Read the model definition and answer for the solid it produces. Units are mm, in the model's axes. A direction names the side the tool comes from. Give positions to 0.01 mm unless a question says otherwise; leave off trailing zeros. Loops run counter-clockwise (first coordinate to the right, second up) from the corner with the lowest first, then second, coordinate; pieces in that order, holes last. Notation, with made-up numbers: (62.25, -35) - (76.25, -35) arc R24 cw to (76.25, -7) - close; hole circle Ø7 at (-7.5, 44.5). An arc over 180 degrees is marked (long way). Use a Markdown table: item, result. Add a question column.
Item 1: For a pull along Y with two mould halves and no side action, classify faces 5 (the face through (7, 0, 2)), 6 (the face through (7, 11, 0)), 7 (the face through (8.475, 4.619, 2.465)) as +Y half, -Y half, draft (parallel to the pull), parting line (faces both ways), or undercut.
Item 2: Each of these flat-tipped pins is pushed along its axis until it touches: P1, Ø7.5, axis at x = 9, y = 8, coming from the -Z side; P2, Ø3, axis at y = 5.5, z = -6.5, coming from the -X side; P3, Ø4, axis at y = 3, z = 3, coming from the -X side; P4, Ø8, axis at y = 7.5, z = -4.5, coming from the +X side. Where does it stop, or does it pass through?
Item 3: A cutting plane is placed at A-A (x = 146.35). Determine the outline of the cut face in (y, z).
Item 4: A cutting plane is placed at D-D (z = -2.5). Determine the outline of the cut face in (x, y), plus the area to 3 significant figures.
Item 5: Consider probe 1 along Y at (x, z) = (146.35, 1.3); probe 2 along X at (y, z) = (14.75, 2); probe 3 along X at (y, z) = (14.5, 3.5). Determine where each line is inside the solid, lowest interval first. Write a range as [from, to].
Item 6: Which of the six approach directions +Z, -Z, +X, -X, +Y, -Y give full straight-line access (tool end or side, diameter ignored) to faces 1 (the face through (15, 17, 3)), 2 (the face through (137.7, 2, 4)), 3 (the face through (75.491, 0.007, -2.17)), 4 (the face through (145, 11, 0))?
Item 7: A cutting plane is placed at C-C (x = 41.5). Determine the outline of the cut face in (y, z), plus the area to 3 significant figures.
Item 8: A cutting plane is placed at B-B (y = 5.5). Determine the outline of the cut face in (x, z), plus the area to 3 significant figures.
from build123d import *

# Parameters (mm, degrees)
SKETCH_W     = 15
SKETCH_H     = 21
SKETCH_R     = 2.3
PAD_DEPTH    = 5
SKETCH001_R  = 7.5
PAD001_DEPTH = 122.7
SKETCH002_W  = 15
SKETCH002_H  = 21
SKETCH002_R  = 2.3
PAD002_DEPTH = 5


with BuildPart() as part:
    # Sketch → Pad (new body)
    with BuildSketch(Plane.XY):
        with Locations((7.5, 10.5)):
            Rectangle(SKETCH_W, SKETCH_H)
        with Locations((6.35, 5.5)):
            Circle(SKETCH_R, mode=Mode.SUBTRACT)
        with Locations((6.35, 15.5)):
            Circle(SKETCH_R, mode=Mode.SUBTRACT)
    extrude(amount=PAD_DEPTH)

    # Sketch001 (on Face2 of Pad) → Pad001 (join)
    with BuildSketch(Plane.YZ.offset(15)):
        with Locations((7.5, -2.5)):
            Circle(SKETCH001_R)
    extrude(amount=PAD001_DEPTH)

    # Sketch002 → Pad002 (join)
    with BuildSketch(Plane.XY):
        with Locations((145.2, 10.5)):
            Rectangle(SKETCH002_W, SKETCH002_H)
        with Locations((146.35, 5.5)):
            Circle(SKETCH002_R, mode=Mode.SUBTRACT)
        with Locations((146.35, 15.5)):
            Circle(SKETCH002_R, mode=Mode.SUBTRACT)
    extrude(amount=PAD002_DEPTH)


solid = part.part
Geometry says:
| question | item | result |
|---|---|---|
| 1 | face 5 | -Y half |
| 1 | face 6 | draft |
| 1 | face 7 | undercut |
| 2 | P1 | z = 0 |
| 2 | P2 | x = 15 |
| 2 | P3 | x = 0 |
| 2 | P4 | x = 137.7 |
| 3 | outline | (0, 0) - (3.2, 0) - (3.2, 5) - (0, 5) - close; (7.8, 0) - (13.2, 0) - (13.2, 5) - (7.8, 5) - close; (17.8, 0) - (21, 0) - (21, 5) - (17.8, 5) - close |
| 4 | outline | (15, 0) - (137.7, 0) - (137.7, 15) - (15, 15) - close |
| 4 | area | 1,840 mm² |
| 5 | probe 1 | [0, 3.2], [7.8, 13.2], [17.8, 21] |
| 5 | probe 2 | [0, 4.18], [8.52, 15], [137.7, 144.18], [148.52, 152.7] |
| 5 | probe 3 | [0, 4.28], [8.42, 15], [137.7, 144.28], [148.42, 152.7] |
| 6 | face 1 | +Z, +Y |
| 6 | face 2 | +Z, -Y |
| 6 | face 3 | none |
| 6 | face 4 | -Z, +X, +Y, -Y |
| 7 | outline | circle Ø15 at (7.5, -2.5) |
| 7 | area | 177 mm² |
| 8 | outline | (0, 0) - (4.05, 0) - (4.05, 5) - (0, 5) - close; (8.65, 0) - (15, 0) - (15, -9.73) - (137.7, -9.73) - (137.7, 0) - (144.05, 0) - (144.05, 5) - (137.7, 5) - (137.7, 4.73) - (15, 4.73) - (15, 5) - (8.65, 5) - close; (148.65, 0) - (152.7, 0) - (152.7, 5) - (148.65, 5) - close |
| 8 | area | 1,880 mm² |
